Drawing for the job (mm, zero at the part's lowest x, y, z). A direction names the side the tool comes from. Give positions to 0.01 mm unless a question says otherwise; leave off trailing zeros. Order: outer loops, then holes, each group sorted by start corner. A loop starts at its lowest first (then second) coordinate and runs counter-clockwise, first axis right, second up. Notation, with made-up numbers: M -28,25.25 L 19,25.25 A4 ccw 19,29.25 Z; hole C 80,45 d3. An arc over 180 degrees is marked long. Answer as a JSON object with one key per item and string values.
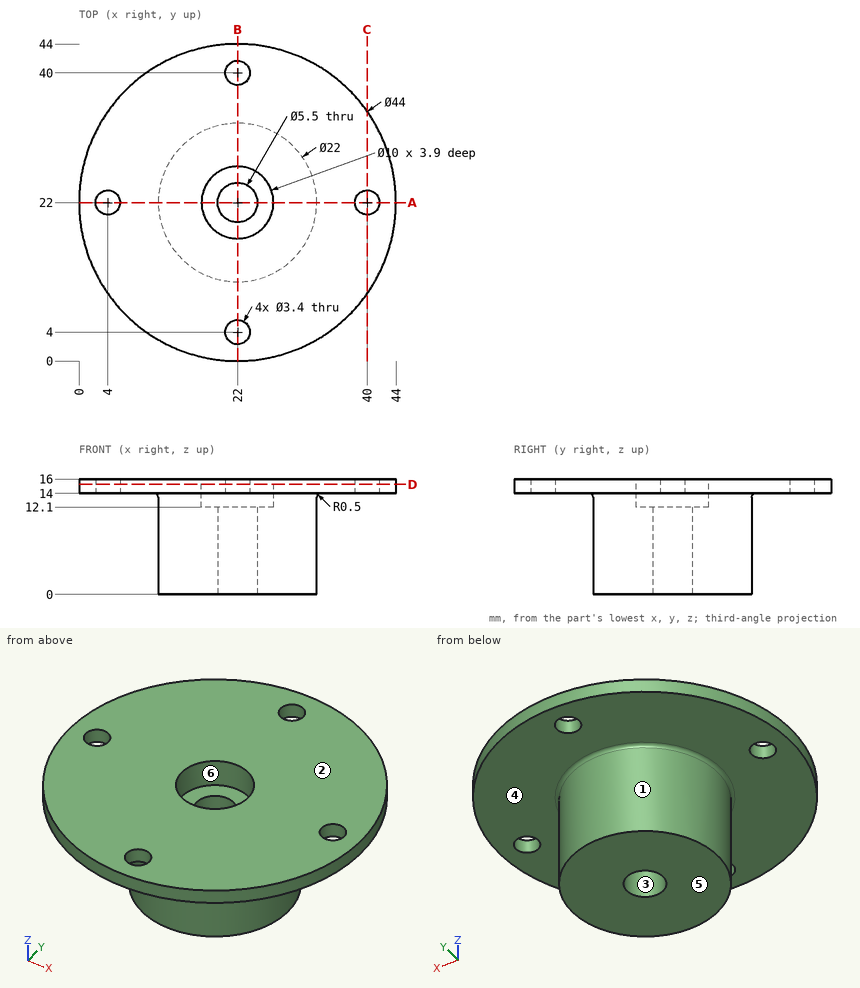
1. Cut at D-D on z = 15.25. Give the cut face in (x, y), plus the area to 3 significant figures.
Worked answers:
{"outline": "C 22,22 d44; hole C 4,22 d3.4; hole C 22,22 d10; hole C 22,4 d3.4; hole C 22,40 d3.4; hole C 40,22 d3.4", "area": "1,410 mm^2"}
2. Probe line 1 along Y through (x, z) = (22, 15); line 2 along Y through (x, z) = (22, 7.5); line 3 along Z through (x, y) = (13.5, 35.5). List the from-to ranges inside material, lowest first.
Worked answers:
{"line 1": "y = 0 to 2.3, 5.7 to 17, 27 to 38.3, 41.7 to 44", "line 2": "y = 11 to 19.25, 24.75 to 33", "line 3": "z = 14 to 16"}
3. Pin check, flat tips, straight feed: P1, Ø2, axis at x = 22, y = 40, coming from the +Z side; P2, Ø4, axis at x = 29.5, y = 28.5, coming from the -Z side; P3, Ø5, axis at x = 18.5, y = 7.5, coming from the -Z side; P4, Ø1.5, axis at y = 30, z = 8.5, coming from the +X side. Stop position of each tip, or through.
Worked answers:
{"P1": "passes through", "P2": "stops at z = 0", "P3": "stops at z = 14", "P4": "stops at x = 30.27"}
4. Two-plate mould, pull along X, no slides. Class the marked faces 1, 2 and 3: +X half, -X half, draft (parallel to the pull), parting line (faces both ways), or undercut.
Worked answers:
{"face 1": "parting line", "face 2": "draft", "face 3": "undercut"}
5. Which spindle directions (+Z, -Z, +X, -X, +Y, -Y) get a long thin tool onto all of the face, cutting with end or side? Do the marked faces 4, 5 and 6. Say none if no direction does.
Worked answers:
{"face 4": "-Z", "face 5": "-Z, +X, -X, +Y, -Y", "face 6": "+Z"}
6. Cut at A-A on y = 22. Give the cut face in (x, z), plus the area to 3 significant figures.
Worked answers:
{"outline": "M 0,14 L 2.3,14 L 2.3,16 L 0,16 Z; M 5.7,14 L 10.5,14 A0.5 cw 11,13.5 L 11,0 L 19.25,0 L 19.25,12.1 L 17,12.1 L 17,16 L 5.7,16 Z; M 24.75,0 L 33,0 L 33,13.5 A0.5 cw 33.5,14 L 38.3,14 L 38.3,16 L 27,16 L 27,12.1 L 24.75,12.1 Z; M 41.7,14 L 44,14 L 44,16 L 41.7,16 Z", "area": "277 mm^2"}
7. Cut at C-C on x = 40. Give the cut face in (y, z).
Worked answers:
{"outline": "M 9.35,14 L 20.3,14 L 20.3,16 L 9.35,16 Z; M 23.7,14 L 34.65,14 L 34.65,16 L 23.7,16 Z"}
